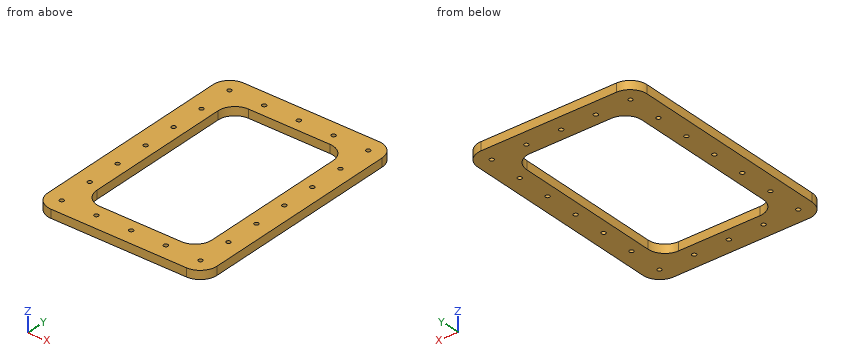
from build123d import *

# Parameters (mm, degrees)
SKETCH1_W           = 100
SKETCH1_H           = 140
SKETCH1_R           = 1.25
SKETCH1_W_2         = 68
SKETCH1_H_2         = 108
BOSS_EXTRUDE1_DEPTH = 5
FILLET1_R           = 10


with BuildPart() as part:
    # Sketch1 → Boss-Extrude1 (new body)
    with BuildSketch(Plane.XY):
        Rectangle(SKETCH1_W, SKETCH1_H)
        with Locations((0, 61)):
            Circle(SKETCH1_R, mode=Mode.SUBTRACT)
        with Locations((-41, 61)):
            Circle(SKETCH1_R, mode=Mode.SUBTRACT)
        with Locations((-20.5, 61)):
            Circle(SKETCH1_R, mode=Mode.SUBTRACT)
        with Locations((20.5, 61)):
            Circle(SKETCH1_R, mode=Mode.SUBTRACT)
        with Locations((41, 61)):
            Circle(SKETCH1_R, mode=Mode.SUBTRACT)
        with Locations((-41, 0)):
            Circle(SKETCH1_R, mode=Mode.SUBTRACT)
        with Locations((-41, 40.666666667)):
            Circle(SKETCH1_R, mode=Mode.SUBTRACT)
        with Locations((-41, 20.333333333)):
            Circle(SKETCH1_R, mode=Mode.SUBTRACT)
        with Locations(Location((41, 40.666666667, 0), (0, 0, 180))):
            Circle(SKETCH1_R, mode=Mode.SUBTRACT)
        with Locations(Location((41, 20.333333333, 0), (0, 0, 180))):
            Circle(SKETCH1_R, mode=Mode.SUBTRACT)
        with Locations(Location((41, 0, 0), (0, 0, 180))):
            Circle(SKETCH1_R, mode=Mode.SUBTRACT)
        with Locations(Location((-20.5, -61, 0), (0, 0, 180))):
            Circle(SKETCH1_R, mode=Mode.SUBTRACT)
        with Locations(Location((0, -61, 0), (0, 0, 180))):
            Circle(SKETCH1_R, mode=Mode.SUBTRACT)
        with Locations(Location((20.5, -61, 0), (0, 0, 180))):
            Circle(SKETCH1_R, mode=Mode.SUBTRACT)
        with Locations(Location((41, -61, 0), (0, 0, 180))):
            Circle(SKETCH1_R, mode=Mode.SUBTRACT)
        with Locations((41, -40.666666667)):
            Circle(SKETCH1_R, mode=Mode.SUBTRACT)
        with Locations((41, -20.333333333)):
            Circle(SKETCH1_R, mode=Mode.SUBTRACT)
        with Locations(Location((-41, -20.333333333, 0), (0, 0, 180))):
            Circle(SKETCH1_R, mode=Mode.SUBTRACT)
        with Locations(Location((-41, -40.666666667, 0), (0, 0, 180))):
            Circle(SKETCH1_R, mode=Mode.SUBTRACT)
        with Locations(Location((-41, -61, 0), (0, 0, 180))):
            Circle(SKETCH1_R, mode=Mode.SUBTRACT)
        Rectangle(SKETCH1_W_2, SKETCH1_H_2, mode=Mode.SUBTRACT)
    extrude(amount=BOSS_EXTRUDE1_DEPTH)

    # Fillet1
    fillet1_edges = [part.edges().sort_by_distance(p)[0] for p in [
        (50, -70, 2.5),
        (-50, -70, 2.5),
        (-50, 70, 2.5),
        (50, 70, 2.5),
        (34, -54, 2.5),
        (34, 54, 2.5),
        (-34, 54, 2.5),
        (-34, -54, 2.5),
    ]]
    fillet(fillet1_edges, radius=FILLET1_R)


solid = part.part
Could you check a few things on this model? Use its own coordinates, in mm. Coordinates: 2 decimals unless noted, no trailing zeros. Order: outer loops, then holes, each group sorted by start corner. A loop starts at its lowest first (then second) coordinate and runs counter-clockwise, first axis right, second up. Notation, with made-up numbers: (41.5, 66) - (69.5, 66) arc R25 cw to (69.5, 82) - close; hole circle Ø1 at (65, 85.5). An arc over 180 degrees is marked (long way). Answer in a Markdown table with one row per item. Add a question column.
(1) I need wall thicknesses on L1, parallel to Y at x = 0, z = 2.5; L2, parallel to X at y = -30.5, z = 0.65; L3, parallel to Y at x = 18, z = 1.25. Which ranges of each line are inside material? Lowest first, please.
(2) If we section it at B-B, the plane x = 10.5: Please give me the cut outline in (y, z), then the cut area to 3 significant figures.
(3) If we section it at A-A, the plane y = 38: Please give me the cut outline in (x, z), then the cut area to 3 significant figures.
(4) If we section it at C-C, the plane z = 1.5: State how many separate pieces and enclosed holes the cut face has, then the cut area to 3 significant figures.
(5) Will this pin go through, and if not, where does the flat tip stop? pin 1 (4 mm diameter, centred on x = -41, y = -20.33, fed in from +Z).
Results are:
| question | item | result |
|---|---|---|
| 1 | L1 | y = -70 to -62.25, -59.75 to -54, 54 to 59.75, 62.25 to 70 |
| 1 | L2 | x = -50 to -34, 34 to 50 |
| 1 | L3 | y = -70 to -54, 54 to 70 |
| 2 | outline | (-70, 0) - (-54, 0) - (-54, 5) - (-70, 5) - close; (54, 0) - (70, 0) - (70, 5) - (54, 5) - close |
| 2 | area | 160 mm2 |
| 3 | outline | (-50, 0) - (-34, 0) - (-34, 5) - (-50, 5) - close; (34, 0) - (50, 0) - (50, 5) - (34, 5) - close |
| 3 | area | 160 mm2 |
| 4 | separate pieces | 1 |
| 4 | enclosed holes | 21 |
| 4 | area | 6,560 mm2 |
| 5 | pin 1 | stops at z = 5 |
